```python
from build123d import *

# Parameters (mm, degrees)
SKETCH1_W               = 25.4
SKETCH1_H               = 19.05
BOSS_EXTRUDE2_DEPTH     = 57.9882
CUT_EXTRUDE3_DEPTH      = 65.019660763
CUT_EXTRUDE3_DEPTH_BACK = 23.8125
SKETCH4_W               = 54.8132
SKETCH4_H               = 17.4625
SKETCH5_R               = 4.0767
CUT_EXTRUDE4_DEPTH      = 23.8125


with BuildPart() as part:
    # Sketch1 → Boss-Extrude2 (new body)
    with BuildSketch(Plane.XY):
        Rectangle(SKETCH1_W, SKETCH1_H)
    extrude(amount=BOSS_EXTRUDE2_DEPTH)

    # Sketch4 → Cut-Extrude3 (cut, two sides: drawn at the far end of the back side and taken through both)
    with BuildSketch(Plane.ZY.offset(12.7).offset(-CUT_EXTRUDE3_DEPTH_BACK)):
        with Locations((28.9941, 0.79375)):
            Rectangle(SKETCH4_W, SKETCH4_H)
    extrude(amount=CUT_EXTRUDE3_DEPTH + CUT_EXTRUDE3_DEPTH_BACK, mode=Mode.SUBTRACT)

    # Sketch5 → Cut-Extrude4 (cut)
    with BuildSketch(Plane(origin=(0, -7.9375, 0), x_dir=(1, 0, 0), z_dir=(0, 1, 0))):
        with Locations(Location((0, -10.054166667, 0), (0, 0, 180))):
            Circle(SKETCH5_R)
        with Locations(Location((0, -49.521533333, 0), (0, 0, 180))):
            Circle(SKETCH5_R)
    extrude(amount=-CUT_EXTRUDE4_DEPTH, mode=Mode.SUBTRACT)


solid = part.part
```
Verification items for the finished model (mm, model axes). A direction names the side the tool comes from. Give positions to 0.01 mm unless a question says otherwise; leave off trailing zeros. Order: outer loops, then holes, each group sorted by start corner. A loop starts at its lowest first (then second) coordinate and runs counter-clockwise, first axis right, second up. Notation, with made-up numbers: (51.5, -23.75) -> (76.5, -23.75) arc R22 ccw to (76.5, -6.75) -> close; hole circle Ø3 at (14.5, 62.5). An arc over 180 degrees is marked (long way). One line per item, written item: value.
(1) Tool access check on faces 1 (the face through (3, -8.72, 52.28)), 2 (the face through (-1, 1, 56.401)). Record the directions out of +Z, -Z, +X, -X, +Y, -Y that give a thin tool (end or side, any length) a straight path to the whole face; none if there is none.
Final values:
face 1: +Y, -Y
face 2: -X, +Y
(2) Sectioned sample at C-C on x = 2. Record the cut outline in (y, z) (1 decimal).
Final values:
outline: (-9.5, 0) -> (9.5, 0) -> (9.5, 1.6) -> (-7.9, 1.6) -> (-7.9, 6.5) -> (-9.5, 6.5) -> close; (-9.5, 13.6) -> (-7.9, 13.6) -> (-7.9, 46) -> (-9.5, 46) -> close; (-9.5, 53.1) -> (-7.9, 53.1) -> (-7.9, 56.4) -> (9.5, 56.4) -> (9.5, 58) -> (-9.5, 58) -> close
(3) Scan lines: line 1 along Z through (x, y) = (0, -8.25); line 2 along Z through (x, y) = (5.5, 4); line 3 along X through (y, z) = (-2.75, 49). Record each from-to range of solid material in increasing order. Write a range as [from, to].
Final values:
line 1: [0, 5.98], [14.13, 45.44], [53.6, 57.99]
line 2: [0, 1.59], [56.4, 57.99]
line 3: [11.11, 12.7]
(4) Sectioned sample at A-A on x = -5.75. Record the cut outline in (y, z) (1 decimal), then the cut area to 4 significant figures.
Final values:
outline: (-9.5, 0) -> (9.5, 0) -> (9.5, 1.6) -> (-7.9, 1.6) -> (-7.9, 56.4) -> (9.5, 56.4) -> (9.5, 58) -> (-9.5, 58) -> close
area: 147.5 mm^2
(5) Gauge pin test, flat ends, axial feed: pin 1 (8.5 mm diameter, centred on y = -1, z = 19, fed in from -X); pin 2 (5 mm diameter, centred on x = 4.5, z = 13.5, fed in from +Y); pin 3 (6.5 mm diameter, centred on x = 0, z = 10.05, fed in from +Y). Record the tip position at first contact, or that the pin passes through.
Final values:
pin 1: x = 11.11
pin 2: y = -7.94
pin 3: through
(6) Sectioned sample at B-B on z = 53. Record the cut outline in (x, y) (1 decimal).
Final values:
outline: (-12.7, -9.5) -> (-2.1, -9.5) -> (-2.1, -7.9) -> (-12.7, -7.9) -> close; (2.1, -9.5) -> (12.7, -9.5) -> (12.7, 9.5) -> (11.1, 9.5) -> (11.1, -7.9) -> (2.1, -7.9) -> close
(7) Sectioned sample at D-D on y = 0.5. Record the cut outline in (x, z), then the cut area to 3 significant figures.
Final values:
outline: (-12.7, 0) -> (12.7, 0) -> (12.7, 57.99) -> (-12.7, 57.99) -> (-12.7, 56.4) -> (11.11, 56.4) -> (11.11, 1.59) -> (-12.7, 1.59) -> close
area: 168 mm^2
(8) Draft check along X on faces 3 (the face through (3.005, -8.72, 12.809)), 4 (the face through (-1, -7.937, 29)), 5 (the face through (12.7, 0, 29)). Enter one of: pulls with the +X half, pulls with the -X half, needs draft (parallel to the pull), parting line crosses it, or undercut.
Final values:
face 3: undercut
face 4: needs draft
face 5: pulls with the +X half
